from build123d import *

# Parameters (mm, degrees)
F0_DEPTH    = 20
F1_T        = -2
F4_D        = 5
F4_ON_F2_D  = 5
F5_SIZE     = 1
F7_T1_DEPTH = 31.2842712475
F7_T3_DEPTH = 23.3408931896


# Not quite as in the source:
# - a fillet or chamfer that OpenCascade refuses, or shapes differently, is made with other operations: its cross-section is extruded or revolved along the edge and cut away or added


with BuildPart() as f0:
    # F6 (on Top) → F0 (new body)
    with BuildSketch(Plane.XY):
        Polygon((-10, -10), (10, -10), (-10, 10), align=None)
    extrude(amount=F0_DEPTH)

    # F1
    f1_openings = [f0.faces().sort_by_distance(p)[0] for p in [
        (0, 0, 10),
    ]]
    offset(amount=F1_T, openings=f1_openings)

    # F4 (through all)
    with Locations(Plane(origin=(0, -8, 0), x_dir=(-1, 0, 0), z_dir=(0, 1, 0))):
        with Locations((0, 10)):
            Hole(F4_D / 2)

    # F4 on F2 (through all)
    with Locations(Plane.YZ.offset(-8)):
        with Locations((0, 10)):
            Hole(F4_ON_F2_D / 2)

    # F5
    f5_edges = [f0.edges().sort_by_distance(p)[0] for p in [
        (-10, 10, 10),
        (10, -10, 10),
    ]]
    chamfer(f5_edges, length=F5_SIZE)

    # F7: fillet of radius 1 on 4 edges, made by hand

    # F7_s2 → F7_t1 (cut)
    with BuildSketch(Plane(origin=(11.0606601718, -11.0606601718, 0), x_dir=(0, 0, 1), z_dir=(-0.7071067812, 0.7071067812, 0))):
        with BuildLine():
            ThreePointArc((0, -1), (0.2928932188, -0.2928932188), (1, 0))
            Line((1, 0), (0, 0))
            Line((0, 0), (0, -1))
        make_face()
        with BuildLine():
            ThreePointArc((20, -1), (19.7071067812, -0.2928932188), (19, 0))
            Line((19, 0), (20, 0))
            Line((20, 0), (20, -1))
        make_face()
    extrude(amount=F7_T1_DEPTH, mode=Mode.SUBTRACT)

    # F7_s4 → F7_t3 (cut)
    with BuildSketch(Plane.XY.offset(-1.6704465948)):
        with BuildLine():
            ThreePointArc((9.0371923242, -9.9102097864), (9.0940980721, -9.3324360321), (8.8204195729, -8.8204195729))
            Line((8.8204195729, -8.8204195729), (9.2928932188, -9.2928932188))
            Line((9.2928932188, -9.2928932188), (9.0371923242, -9.9102097864))
        make_face()
        with BuildLine():
            ThreePointArc((-8.8204195729, 8.8204195729), (-9.3324360321, 9.0940980721), (-9.9102097864, 9.0371923242))
            Line((-9.9102097864, 9.0371923242), (-9.2928932188, 9.2928932188))
            Line((-9.2928932188, 9.2928932188), (-8.8204195729, 8.8204195729))
        make_face()
    extrude(amount=F7_T3_DEPTH, mode=Mode.SUBTRACT)


solid = f0.part
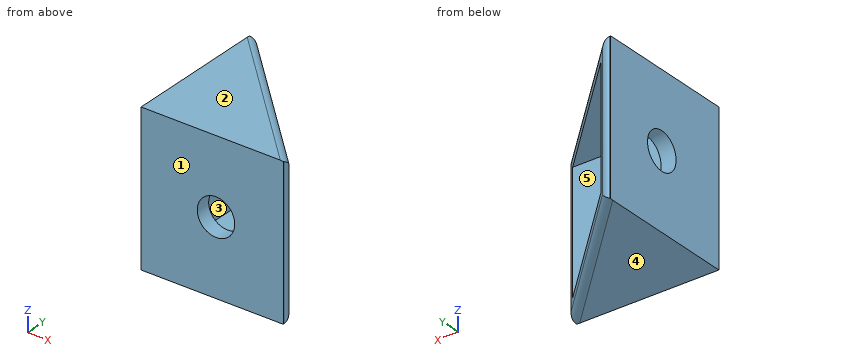
Check sheet for the modelled part. Datum: model origin and axes. Units: mm. Face numbers are marked on the shaded views. A direction names the side the tool comes from. Round coordinates to 2 decimals unless told otherwise and drop trailing zeros. Order: outer loops, then holes, each group sorted by start corner. A loop starts at its lowest first (then second) coordinate and runs counter-clockwise, first axis right, second up.
Q1. Cross-section at A-A, the plane z = 10. Enter the section's corners in (x, y).
Filled sheet:
outline: (-10, -10) - (-2.5, -10) - (-2.5, -8) - (-8, -8) - (-8, -2.5) - (-10, -2.5) - close; (-10, 2.5) - (-8, 2.5) - (-8, 8) - (-8.82, 8.82) arc R1 ccw to (-9.91, 9.04) - (-10, 9) - close; (2.5, -10) - (9, -10) - (9.04, -9.91) arc R1 ccw to (8.82, -8.82) - (8, -8) - (2.5, -8) - close
Q2. Depth check by flat-ended pin: P1, Ø6, axis at x = -1, y = 5.5, coming from the -Z side; P2, Ø8, axis at y = 2.5, z = 11.5, coming from the +X side; P3, Ø5, axis at x = 0.5, y = 2.5, coming from the -Z side. Enter the tip coordinate at first touch or a pass-through.
Filled sheet:
P1: passes through
P2: stops at x = -8
P3: stops at z = 0.22
Q3. Cross-section at B-B, the plane z = 5. Enter the section's corners in (x, y), plus the area to 3 significant figures.
Filled sheet:
outline: (-10, -10) - (9, -10) - (9.04, -9.91) arc R1 ccw to (8.82, -8.82) - (8, -8) - (-8, -8) - (-8, 8) - (-8.82, 8.82) arc R1 ccw to (-9.91, 9.04) - (-10, 9) - close
area: 71.1 mm2
Q4. Scan lines: L1, parallel to Z at x = -9.05, y = 0; L2, parallel to Z at x = -1.5, y = -5.25; L3, parallel to X at y = -6, z = 17. Record each from-to range of solid material in increasing order.
Filled sheet:
L1: z = 0 to 7.5, 12.5 to 20
L2: z = 0 to 2, 18 to 20
L3: x = -10 to -8
Q5. Set-up check for the marked faces 4 and 5: record each of +Z, -Z, +X, -X, +Y, -Y from which the full face is reachable in a straight line by a thin tool's end or side.
Filled sheet:
face 4: -Z, +X, -X, +Y, -Y
face 5: +X, +Y
Q6. Draft check along Z on the marked faces 1, 2 and 3. Enter one of: pulls with the +Z half, pulls with the -Z half, needs draft (parallel to the pull), parting line crosses it, or undercut.
Filled sheet:
face 1: needs draft
face 2: pulls with the +Z half
face 3: undercut
